Part model, mm, in its own coordinate system. Round coordinates to 2 decimals unless told otherwise and drop trailing zeros. Write each loop counter-clockwise with the first axis right and the second up, starting at its lowest first coordinate (ties: lowest second). Pieces come first, ordered by that corner, then holes.
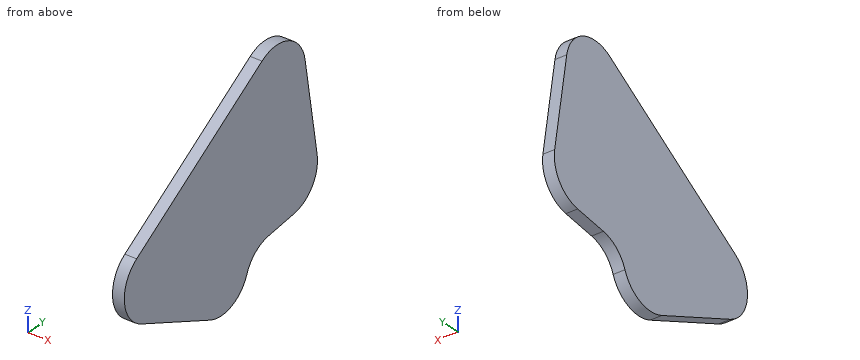
```python
from build123d import *

# Parameters (mm, degrees)
BOSS_EXTRUDE1_START = 66.421062
BOSS_EXTRUDE1_DEPTH = 3.175
FILLET1_R           = 9.525


with BuildPart() as part:
    # Sketch1 → Boss-Extrude1 (new body)
    with BuildSketch(Plane(origin=(0, 0, 0), x_dir=(0, 0, -1), z_dir=(1, 0, 0)).offset(BOSS_EXTRUDE1_START)):
        with BuildLine():
            Line((-1123.745691864, 290.969312893), (-1113.943201538, 314.401580889))
            ThreePointArc((-1113.943201538, 314.401580889), (-1115.256946713, 323.982985548), (-1124.274989939, 327.476427692))
            Line((-1124.274989939, 327.476427692), (-1124.257483159, 327.479304887))
            Line((-1124.257483159, 327.479304887), (-1126.831962996, 343.144159772))
            ThreePointArc((-1126.831962996, 343.144159772), (-1130.677100149, 349.33776623), (-1137.77556383, 350.998384801))
            Line((-1137.77556383, 350.998384801), (-1162.839331646, 346.879217061))
            ThreePointArc((-1162.839331646, 346.879217061), (-1170.036672625, 341.262176157), (-1169.202400053, 332.170594614))
            Line((-1169.202400053, 332.170594614), (-1140.440548672, 289.335537249))
            ThreePointArc((-1140.440548672, 289.335537249), (-1131.605097766, 285.165531172), (-1123.745691864, 290.969312893))
        make_face()
    extrude(amount=BOSS_EXTRUDE1_DEPTH)

    # Fillet1
    # the kernel refuses this fillet: 9.525 mm, written as the material it adds along each edge
    with BuildSketch(Plane(origin=(66.421062, 327.476427692, 1124.274989939), x_dir=(0, -0.5830735725589627, -0.8124193553721674), z_dir=(1, 0, 0))) as fillet1_piece_1_section:
        with BuildLine():
            CenterArc((20.205576272, 6.735192091), FILLET1_R, 135, 90)
            Line((13.470384182, 13.470384182), (0, 0))
            ThreePointArc((0, 0), (6.735192091, 2.789807909), (13.470384182, 0))
        make_face()
    fillet1_piece_1 = extrude(amount=3.175, mode=Mode.PRIVATE)
    fillet1_piece_1 = split(fillet1_piece_1, bisect_by=Plane(origin=(68.008562, 327.479299996, 1124.257482355), z_dir=(0, -0.1621719582624188, 0.9867625124381917)), keep=Keep.TOP, mode=Mode.PRIVATE)
    add(fillet1_piece_1)
    # the kernel refuses this fillet: 9.525 mm, written as the material it adds along each edge
    with BuildSketch(Plane(origin=(69.596062, 327.479288583, 1124.257480479), x_dir=(0, 0.9867625124381958, 0.162171958262393), z_dir=(-1, 0, 0))) as fillet1_2_piece_1:
        with BuildLine():
            CenterArc((6.9625446, 9.525), FILLET1_R, 210.061634747, 59.938365253)
            ThreePointArc((-1.281219438, 4.753629183), (-0.328171819, 2.461024254), (0, 0))
            Line((0, 0), (6.9625446, 0))
        make_face()
    extrude(amount=3.175)


solid = part.part
```
Q1. Cut at C-C on y = 306. Write the cut outline in (x, z), plus the area to 3 significant figures.
Values follow:
outline: (66.42, 1117.46) - (69.6, 1117.46) - (69.6, 1151.63) - (66.42, 1151.63) - close
area: 108 mm2
Q2. Cut at A-A on x = 67.45. Write the cut outline in (y, z) (3 decimals).
Values follow:
outline: (289.336, 1140.441) arc R9.525 ccw to (290.969, 1123.746) - (314.402, 1113.943) arc R9.525 ccw to (326.986, 1119.359) arc R9.525 cw to (334.35, 1125.387) - (343.144, 1126.832) arc R9.525 ccw to (350.998, 1137.776) - (346.879, 1162.839) arc R9.525 ccw to (332.171, 1169.202) - close
Q3. Cut at B-B on z = 1149. Write the cut outline in (x, y), plus the area to 3 significant figures.
Values follow:
outline: (66.42, 302.08) - (69.6, 302.08) - (69.6, 349.15) - (66.42, 349.15) - close
area: 149 mm2
Q4. Wall check: L1, parallel to Y at x = 67.65, z = 1136; L2, parallel to Z at x = 69.25, y = 289; L3, parallel to Y at x = 68.6, z = 1122. Give the ranges that are in metal, low to high.
Values follow:
L1: y = 285.77 to 351.12
L2: z = 1124.86 to 1140.2
L3: y = 295.14 to 328.51
Q5. Drop a flat-ended pin along its axis: pin 1 (1 mm diameter, centred on x = 69, z = 1137, fed in from -Y). Give the stop position or say it passes through.
Values follow:
pin 1: stops at y = 285.99
